The listing builds one solid part. Answer for the finished solid, in the listing's coordinates (mm). Face numbers are marked on the shaded views. Coordinates: 2 decimals unless noted, no trailing zeros.
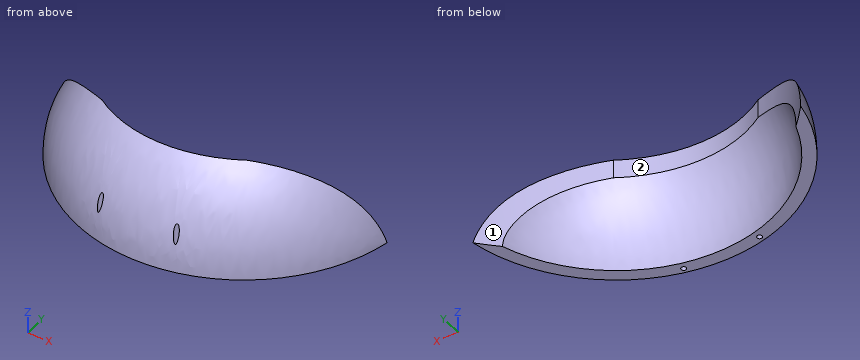
from build123d import *

# Parameters (mm, degrees)
PAD_DEPTH        = 55
REVOLUTION_ANGLE = -90
SKETCH002_R      = 1
POCKET_DEPTH     = 38.367652


with BuildPart() as pad:
    # Sketch001 → Pad (new body)
    with BuildSketch(Plane.XY):
        with BuildLine():
            ThreePointArc((-28.678822, -28.957602), (0, -38), (28.678822, -28.957602))
            ThreePointArc((28.678822, -28.957602), (47.930354, -15.847158), (65, 0))
            Line((-65, 0), (65, 0))
            ThreePointArc((-65, 0), (-48.373276, -16.40271), (-28.678822, -28.957602))
        make_face()
    extrude(amount=PAD_DEPTH)


with BuildPart() as holesscrews:
    # Sketch → Revolution (revolve)
    with BuildSketch(Plane.XY):
        with BuildLine():
            ThreePointArc((-59.808026, 0), (0, -49), (59.808026, 0))
            Line((59.808026, 0), (64.899923, 0))
            ThreePointArc((-64.899923, 0), (0, -54), (64.899923, 0))
            Line((-64.899923, 0), (-59.808026, 0))
        make_face()
    revolve(axis=Axis((0, 0, 0), (1, 0, 0)), revolution_arc=REVOLUTION_ANGLE)

    # Cut: cut Pad
    add(pad.part, mode=Mode.SUBTRACT)

    # Sketch002 → Pocket (cut, through all)
    with BuildSketch(Plane(origin=(0, 0, 0), x_dir=(1, 0, 0), z_dir=(0, 0, -1))):
        with Locations((15.028955, 50.094116)):
            Circle(SKETCH002_R)
        with Locations((-15.028955, 50.094116)):
            Circle(SKETCH002_R)
    extrude(amount=-POCKET_DEPTH, mode=Mode.SUBTRACT)


solid = holesscrews.part
Q1. Given pin 1 (8 mm diameter, centred on y = -6.5, z = 10.5, fed in from +X); pin 2 (12 mm diameter, centred on x = -4.5, y = -40, fed in from +Z); pin 3 (5 mm diameter, centred on x = -5.5, y = -44.5, fed in from +Z); pin 4 (1.5 mm diameter, centred on y = -13, z = 7.5, fed in from +X), each flat-ended and moving along its own axis, determine where each tip first touches the part or whether it passes through.
Answers below:
pin 1: stops at x = 62.78
pin 2: stops at z = 38.37
pin 3: stops at z = 33.59
pin 4: stops at x = 60.55
Q2. The part is cut by section A-A, the plane z = 5. State how many separate pieces and enclosed holes the cut face has, then the cut area to 3 significant figures.
Answers below:
separate pieces: 1
enclosed holes: 2
area: 821 mm2
Q3. Determine the mould class of the marked faces 1 and 2 for opening direction X: released by +X, released by -X, zero draft, split by the parting line, or undercut.
Answers below:
face 1: undercut
face 2: undercut
Q4. Find the intervals of material crossed by probe 1 along X at (y, z) = (-17.5, 13.5); probe 2 along X at (y, z) = (-30.5, 18); probe 3 along Y at (x, z) = (-22.5, 17.5), in increasing order.
Answers below:
probe 1: x = -56.51 to -50.58, 50.58 to 56.51
probe 2: x = -45.91 to -38.38, 38.38 to 45.91
probe 3: y = -46.89 to -41.13
